Source: CAD feature listing. Evaluate the final solid. Frame: model axes, mm. Give positions to 0.01 mm unless a question says otherwise; leave off trailing zeros. Order: outer loops, then holes, each group sorted by start corner. A loop starts at its lowest first (then second) coordinate and runs counter-clockwise, first axis right, second up. Notation, with made-up numbers: (19, 46.25) -> (69, 46.25) arc R22 cw to (69, 65.25) -> close; hole circle Ø1 at (-4, 79.5). An arc over 180 degrees is marked (long way). Use CSV: the item, a comma, the result in double quotes.
```python
from build123d import *

# Parameters (mm, degrees)
SKETCH_R  = 1.1
PAD_DEPTH = 16


with BuildPart() as part:
    # Sketch → Pad (new body)
    with BuildSketch(Plane.XZ):
        Polygon((-1.59, -2.753961), (1.59, -2.753961), (3.18, 0), (1.59, 2.753961), (-1.59, 2.753961), (-3.18, 0), align=None)
        Circle(SKETCH_R, mode=Mode.SUBTRACT)
    extrude(amount=PAD_DEPTH)


solid = part.part
```
1. Mould query, pull axis Z, two halves, no side actions, for faces 1 (the cylindrical face through (1.05, -7.89, 0.33)), 2 (the flat face through (-2.37, -7.89, 1.4)), 3 (the flat face through (1.4, 0, 0)). Classes: released by +Z, released by -Z, zero draft, split by the parting line, or undercut.
Answer below:
face 1,"undercut"
face 2,"released by +Z"
face 3,"zero draft"
2. Section query D-D on x = 2.5. Return loops of the section in (y, z).
Answer below:
outline,"(-16, -1.18) -> (0, -1.18) -> (0, 1.18) -> (-16, 1.18) -> close"
3. Section query A-A on x = 0. Return loops of the section in (y, z), plus the area to 3 significant figures.
Answer below:
outline,"(-16, -2.75) -> (0, -2.75) -> (0, -1.1) -> (-16, -1.1) -> close; (-16, 1.1) -> (0, 1.1) -> (0, 2.75) -> (-16, 2.75) -> close"
area,"52.9 mm²"
4. Pin query (flat end, axial travel): P1, Ø1, axis at x = 1.5, z = 1, coming from the +Y side. Return the tip coordinate at first contact, or that it passes through.
Answer below:
P1,"stops at y = 0"
5. Ray query, line 1 along Z through (x, y) = (0, -6.5); line 2 along X through (y, z) = (-11.75, 0.85); line 3 along X through (y, z) = (-0.25, 0.4). Return the intervals inside material, ascending.
Answer below:
line 1,"z = -2.75 to -1.1, 1.1 to 2.75"
line 2,"x = -2.69 to -0.7, 0.7 to 2.69"
line 3,"x = -2.95 to -1.02, 1.02 to 2.95"
6. Section query C-C on y = -3.5. Return loops of the section in (x, z).
Answer below:
outline,"(-3.18, 0) -> (-1.59, -2.75) -> (1.59, -2.75) -> (3.18, 0) -> (1.59, 2.75) -> (-1.59, 2.75) -> close; hole circle Ø2.2 at (0, 0)"
7. Section query B-B on z = 0.3. Return loops of the section in (x, y).
Answer below:
outline,"(-3.01, -16) -> (-1.06, -16) -> (-1.06, 0) -> (-3.01, 0) -> close; (1.06, -16) -> (3.01, -16) -> (3.01, 0) -> (1.06, 0) -> close"
